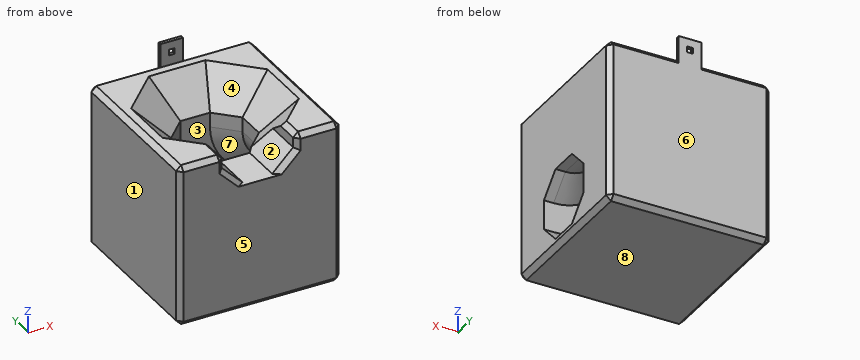
from build123d import *

# Parameters (mm, degrees)
SKETCH1_W                = 50
SKETCH1_H                = 50
BOSS_EXTRUDE1_DEPTH      = 50
CHAMFER1_SIZE            = 10
CUT_EXTRUDE1_DEPTH       = 22
CHAMFER2_SIZE            = 1.5
BOSS_EXTRUDE2_DEPTH      = 7
BOSS_EXTRUDE2_DEPTH_BACK = 10
SKETCH11_W               = 7
SKETCH11_H               = 1
SKETCH12_W               = 1.8
SKETCH12_H               = 1.8
CUT_EXTRUDE2_DEPTH       = 7


with BuildPart() as part:
    # Sketch1 → Boss-Extrude1 (new body)
    with BuildSketch(Plane.XY):
        with Locations((25, 25)):
            Rectangle(SKETCH1_W, SKETCH1_H)
    extrude(amount=BOSS_EXTRUDE1_DEPTH)

    # Cut-Sweep5: sweep along a path in Sketch9
    with BuildLine(Plane(origin=(0, 25, 0), x_dir=(-1, 0, 0), z_dir=(0, -1, 0))) as cut_sweep5_path:
        Line((-50, -13.5), (-47, -13.5))
        ThreePointArc((-47, -13.5), (-31.443650814, -19.943650814), (-25, -35.5))
        Line((-25, -35.5), (-25, -50))
    # Sketch8 → Cut-Sweep5 (sweep, cut)
    with BuildSketch(Plane(origin=(50, 0, 0), x_dir=(0, 0, -1), z_dir=(1, 0, 0))):
        Polygon((-2.5, 29.556349186), (-8.943650814, 36), (-18.056349186, 36), (-24.5, 29.556349186), (-24.5, 20.443650814), (-18.056349186, 14), (-8.943650814, 14), (-2.5, 20.443650814), align=None)
    sweep(path=cut_sweep5_path.line, mode=Mode.SUBTRACT)

    # Chamfer1
    chamfer1_edges = [part.edges().sort_by_distance(p)[0] for p in [
        (17.221825407, 17.221825407, 50),
        (32.778174593, 17.221825407, 50),
        (36, 25, 50),
        (32.778174593, 32.778174593, 50),
        (17.221825407, 32.778174593, 50),
        (14, 25, 50),
        (25, 14, 50),
        (25, 36, 50),
    ]]
    chamfer(chamfer1_edges, length=CHAMFER1_SIZE)

    # Sketch10 → Cut-Extrude1 (cut)
    with BuildSketch(Plane.XZ):
        Polygon((29.556349186, 39), (36, 45.443650814), (36, 54.556349186), (29.556349186, 61), (20.443650814, 61), (14, 54.556349186), (14, 45.443650814), (20.443650814, 39), align=None)
    extrude(amount=-CUT_EXTRUDE1_DEPTH, mode=Mode.SUBTRACT)

    # Chamfer2
    chamfer2_edges = [part.edges().sort_by_distance(p)[0] for p in [
        (50, 25, 50),
        (25, 50, 50),
        (0, 25, 50),
        (25, 50, 0),
        (50, 25, 0),
        (25, 0, 0),
        (0, 25, 0),
        (7, 0, 50),
        (0, 50, 25),
        (50, 50, 25),
        (50, 0, 25),
        (0, 0, 25),
        (43, 0, 50),
        (36, 0, 47.721825407),
        (14, 0, 47.721825407),
        (17.221825407, 0, 42.221825407),
        (32.778174593, 0, 42.221825407),
        (14, 3.150757595, 50),
        (36, 3.150757595, 50),
    ]]
    chamfer(chamfer2_edges, length=CHAMFER2_SIZE)

    # Sketch11 → Boss-Extrude2 (add, two sides: drawn at the far end of the back side and taken through both)
    with BuildSketch(Plane.XY.offset(50).offset(-BOSS_EXTRUDE2_DEPTH_BACK)):
        with Locations((25, 49.5)):
            Rectangle(SKETCH11_W, SKETCH11_H)
    extrude(amount=BOSS_EXTRUDE2_DEPTH + BOSS_EXTRUDE2_DEPTH_BACK)

    # Sketch12 → Cut-Extrude2 (cut)
    with BuildSketch(Plane.XZ.offset(-49)):
        with Locations((25, 53.6)):
            Rectangle(SKETCH12_W, SKETCH12_H)
    extrude(amount=-CUT_EXTRUDE2_DEPTH, mode=Mode.SUBTRACT)


solid = part.part
Verification items for the finished model (mm, model axes). Face numbers are marked on the shaded views. A direction names the side the tool comes from. Coordinates: 2 decimals unless noted, no trailing zeros. Write each loop counter-clockwise with the first axis right and the second up, starting at its lowest first coordinate (ties: lowest second). Pieces come first, ordered by that corner, then holes. Notation, with made-up numbers: (31, 14.25) - (86, 14.25) arc R24 cw to (86, 45.25) - close; hole circle Ø7 at (-24.5, 34). An arc over 180 degrees is marked (long way). Answer as a JSON object with one key per item and string values.
(1) Cross-section at C-C on x = 6. Record the cut outline in (y, z).
Report:
{"outline": "(0, 1.5) - (1.5, 0) - (48.5, 0) - (50, 1.5) - (50, 48.5) - (48.5, 50) - (35.7, 50) - (32.87, 48) - (17.13, 48) - (14.3, 50) - (1.5, 50) - (0, 48.5) - close"}
(2) Cross-section at A-A on y = 34.5. Record the cut outline in (x, z).
Report:
{"outline": "(0, 1.5) - (1.5, 0) - (48.5, 0) - (50, 1.5) - (50, 7.44) - (47, 7.44) arc R28.06 cw to (18.94, 35.5) - (18.94, 40) - (4.8, 50) - (1.5, 50) - (0, 48.5) - close; (31.06, 35.5) arc R15.94 ccw to (47, 19.56) - (50, 19.56) - (50, 48.5) - (48.5, 50) - (45.2, 50) - (31.06, 40) - close"}
(3) Tool access check on the marked faces 1, 2, 3 and 4. Record the directions out of +Z, -Z, +X, -X, +Y, -Y that give a thin tool (end or side, any length) a straight path to the whole face; none if there is none.
Report:
{"face 1": "+Z, -Z, -X, +Y, -Y", "face 2": "+Z, -Y", "face 3": "none", "face 4": "+Z"}
(4) Cross-section at B-B on z = 42. Record the cut outline in (x, y), plus the area to 3 significant figures.
Report:
{"outline": "(0, 1.5) - (1.5, 0) - (15.32, 0) - (17.44, 1.5) - (17.44, 14.17) - (12, 19.62) - (12, 30.38) - (19.62, 38) - (30.38, 38) - (38, 30.38) - (38, 19.62) - (32.56, 14.17) - (32.56, 1.5) - (34.68, 0) - (48.5, 0) - (50, 1.5) - (50, 48.5) - (48.5, 50) - (1.5, 50) - (0, 48.5) - close", "area": "1,750 mm^2"}
(5) Mould release check, pull along Y, two halves, no side actions. Record for the marked faces 5, 6, 7 and 8: pulls with the +Y half, pulls with the -Y half, needs draft (parallel to the pull), parting line crosses it, or undercut.
Report:
{"face 5": "pulls with the -Y half", "face 6": "pulls with the +Y half", "face 7": "undercut", "face 8": "needs draft"}
(6) Thickness scan on line 1 along X through (y, z) = (19.5, 8); line 2 along Y through (x, z) = (44, 9.5); line 3 along Y through (x, z) = (40, 46). Record the ranges inside material, lowest first.
Report:
{"line 1": "0 to 30.53", "line 2": "0 to 14, 36 to 50", "line 3": "0 to 15.96, 34.04 to 50"}
(7) Gauge pin test, flat ends, axial feed: pin 1 Ø0.8 at (y, z) = (49.5, 52.5) entering from -X; pin 2 Ø5.5 at (x, z) = (25.5, 52) entering from -Y; pin 3 Ø14 at (x, y) = (35, 22.5) entering from +Z. Record the tip position at first contact, or that the pin passes through.
Report:
{"pin 1": "x = 21.5", "pin 2": "y = 45.25", "pin 3": "z = 46"}
(8) Cross-section at D-D on y = 41. Record the cut outline in (x, z), plus the area to 3 significant figures.
Report:
{"outline": "(0, 1.5) - (1.5, 0) - (48.5, 0) - (50, 1.5) - (50, 48.5) - (48.5, 50) - (38.7, 50) - (31.63, 45) - (18.37, 45) - (11.3, 50) - (1.5, 50) - (0, 48.5) - close", "area": "2,390 mm^2"}
